```python
from build123d import *

# Parameters (mm, degrees)
F0_R     = 63.5
F1_DEPTH = 101.6
F2_W     = 57.8431412578
F2_H     = 53.4668527544
F3_DEPTH = 190.5
F4_R     = 2.54
F5_R     = 7.6327
F6_DEPTH = 57.912


with BuildPart() as f1:
    # F0 (on Top) → F1 (new body)
    with BuildSketch(Plane.XY):
        Circle(F0_R)
    extrude(amount=F1_DEPTH)

    # F2 (on face) → F3 (cut)
    with BuildSketch(Plane.XY.offset(101.6)):
        Rectangle(F2_W, F2_H)
    extrude(amount=-F3_DEPTH, mode=Mode.SUBTRACT)

    # F4
    f4_edges = [f1.edges().sort_by_distance(p)[0] for p in [
        (-63.5, 0, 101.6),
        (0, -26.733426, 101.6),
        (28.921571, 0, 101.6),
        (0, 26.733426, 101.6),
        (-28.921571, 0, 101.6),
    ]]
    fillet(f4_edges, radius=F4_R)

    # F5 (on face) → F6 (cut)
    with BuildSketch(Plane.YZ.offset(-28.9215706289)):
        with Locations((0, 52.9904067516)):
            Circle(F5_R)
    extrude(amount=-F6_DEPTH, mode=Mode.SUBTRACT)


solid = f1.part
```
CAD build for the part. Positions are in the model's coordinates, mm. A direction names the side the tool comes from. Round coordinates to 2 decimals unless told otherwise and drop trailing zeros. Order: outer loops, then holes, each group sorted by start corner. A loop starts at its lowest first (then second) coordinate and runs counter-clockwise, first axis right, second up.
Item 1: Pin check, flat tips, straight feed: pin 1 (12 mm diameter, centred on y = 48, z = 59.5, fed in from -X); pin 2 (1 mm diameter, centred on y = -21, z = 47.5, fed in from -X); pin 3 (10 mm diameter, centred on y = -39, z = 37, fed in from +X). Stop position of each tip, or through.
Item 2: Mould opens along X. For faces 1 (the face through (0, 26.733, 50)), 2 (the face through (58.66, -24.32, 48.84)), 3 (the face through (-1, -27, 0)) say: pulls with the +X half, pulls with the -X half, needs draft (parallel to the pull), parting line crosses it, or undercut.
Item 3: Saw through at B-B on x = 0. Write the cut outline in (y, z).
Item 4: Saw through at C-C on z = 73.5. Write the cut outline in (x, y).
Item 5: Probe line 1 along Z through (x, y) = (-55, 0); line 2 along Y through (x, z) = (-4, 5.5); line 3 along Y through (x, z) = (-19, 78.5). List the from-to ranges inside material, lowest first.
Item 6: Tool access for faces 4 (the face through (-1, -40, 101.6)), 5 (the face through (0, -26.733, 50)), 6 (the face through (-45.97, -0.99, 60.56)): list every direction of +Z, -Z, +X, -X, +Y, -Y with a clear straight run to the whole face (end or side of a thin tool).
Item 7: Saw through at A-A on y = 0. Write the cut outline in (x, z), then the cut area to 3 significant figures.
Reported:
1. pin 1: stops at x = -47.63
1. pin 2: stops at x = -60.1
1. pin 3: stops at x = 53.63
2. face 1: undercut
2. face 2: parting line crosses it
2. face 3: needs draft
3. outline: (-63.5, 0) - (-26.73, 0) - (-26.73, 99.06) arc R2.54 ccw to (-29.27, 101.6) - (-60.96, 101.6) arc R2.54 ccw to (-63.5, 99.06) - close; (26.73, 0) - (63.5, 0) - (63.5, 99.06) arc R2.54 ccw to (60.96, 101.6) - (29.27, 101.6) arc R2.54 ccw to (26.73, 99.06) - close
4. outline: circle Ø127 at (0, 0); hole (-28.92, -26.73) - (28.92, -26.73) - (28.92, 26.73) - (-28.92, 26.73) - close
5. line 1: z = 0 to 45.36, 60.62 to 101.6
5. line 2: y = -63.37 to -26.73, 26.73 to 63.37
5. line 3: y = -60.59 to -26.73, 26.73 to 60.59
6. face 4: +Z, +X, -X, +Y, -Y
6. face 5: +Z, -Z
6. face 6: -X
7. outline: (-63.5, 0) - (-28.92, 0) - (-28.92, 45.36) - (-63.5, 45.36) - close; (-63.5, 60.62) - (-28.92, 60.62) - (-28.92, 99.06) arc R2.54 ccw to (-31.46, 101.6) - (-60.96, 101.6) arc R2.54 ccw to (-63.5, 99.06) - close; (28.92, 0) - (63.5, 0) - (63.5, 99.06) arc R2.54 ccw to (60.96, 101.6) - (31.46, 101.6) arc R2.54 ccw to (28.92, 99.06) - close
7. area: 6,490 mm2
